from build123d import *

# Parameters (mm, degrees)
SKETCH1_W           = 120
SKETCH1_H           = 110
BOSS_EXTRUDE1_DEPTH = 2.5
SKETCH2_R           = 14.5
CUT_EXTRUDE1_DEPTH  = 4
SKETCH3_R           = 20
CUT_EXTRUDE2_DEPTH  = 10
SKETCH5_R           = 1.6
CUT_EXTRUDE5_DEPTH  = 10
CUT_EXTRUDE6_DEPTH  = 10
SKETCH8_W           = 5
SKETCH8_H           = 10
SKETCH8_W_2         = 10
SKETCH8_H_2         = 5
BOSS_EXTRUDE2_DEPTH = 14
SKETCH9_R           = 1.5
CUT_EXTRUDE7_DEPTH  = 120.910383203
SKETCH10_R          = 1.5
CUT_EXTRUDE8_DEPTH  = 5
FILLET1_R           = 2.5


with BuildPart() as part:
    # Sketch1 → Boss-Extrude1 (new body)
    with BuildSketch(Plane(origin=(0, 0, 0), x_dir=(1, 0, 0), z_dir=(0, 1, 0))):
        Rectangle(SKETCH1_W, SKETCH1_H)
    extrude(amount=BOSS_EXTRUDE1_DEPTH)

    # Sketch2 → Cut-Extrude1 (cut)
    with BuildSketch(Plane(origin=(0, 2.5, 0), x_dir=(1, 0, 0), z_dir=(0, 1, 0))):
        with Locations(Location((40, 30, 0), (0, 0, 270))):
            Circle(SKETCH2_R)
        with Locations(Location((10, 30, 0), (0, 0, 270))):
            Circle(SKETCH2_R)
        with Locations(Location((-40, -5, 0), (0, 0, 270))):
            Circle(SKETCH2_R)
        with Locations(Location((-40, -35, 0), (0, 0, 270))):
            Circle(SKETCH2_R)
    extrude(amount=-CUT_EXTRUDE1_DEPTH, mode=Mode.SUBTRACT)

    # Sketch3 → Cut-Extrude2 (cut)
    with BuildSketch(Plane(origin=(0, 2.5, 0), x_dir=(1, 0, 0), z_dir=(0, 1, 0))):
        with Locations(Location((25, -20, 0), (0, 0, 270))):
            Circle(SKETCH3_R)
    extrude(amount=-CUT_EXTRUDE2_DEPTH, mode=Mode.SUBTRACT)

    # Sketch5 → Cut-Extrude5 (cut)
    with BuildSketch(Plane(origin=(0, 2.5, 0), x_dir=(1, 0, 0), z_dir=(0, 1, 0))):
        with Locations(Location((-56, 51, 0), (0, 0, 270))):
            Circle(SKETCH5_R)
        with Locations(Location((56, 51, 0), (0, 0, 270))):
            Circle(SKETCH5_R)
        with Locations(Location((56, -51, 0), (0, 0, 270))):
            Circle(SKETCH5_R)
        with Locations(Location((-56, -51, 0), (0, 0, 270))):
            Circle(SKETCH5_R)
    extrude(amount=-CUT_EXTRUDE5_DEPTH, mode=Mode.SUBTRACT)

    # Sketch7 → Cut-Extrude6 (cut)
    with BuildSketch(Plane(origin=(0, 2.5, 0), x_dir=(1, 0, 0), z_dir=(0, 1, 0))):
        with BuildLine():
            Line((-54.5, -5), (-54.5, 0))
            ThreePointArc((-54.5, 0), (-40, 14.5), (-25.5, 0))
            Line((-25.5, 0), (-25.5, -5))
            ThreePointArc((-25.5, -5), (-40, -19.5), (-54.5, -5))
        make_face()
        with BuildLine():
            Line((10, 15.5), (5, 15.5))
            ThreePointArc((5, 15.5), (-9.5, 30), (5, 44.5))
            Line((5, 44.5), (10, 44.5))
            ThreePointArc((10, 44.5), (24.5, 30), (10, 15.5))
        make_face()
    extrude(amount=-CUT_EXTRUDE6_DEPTH, mode=Mode.SUBTRACT)

    # Sketch8 → Boss-Extrude2 (add)
    with BuildSketch(Plane(origin=(0, 2.5, 0), x_dir=(1, 0, 0), z_dir=(0, 1, 0))):
        with Locations((-17.5, -20)):
            Rectangle(SKETCH8_W, SKETCH8_H)
        with Locations((25, 50)):
            Rectangle(SKETCH8_W_2, SKETCH8_H_2)
    extrude(amount=BOSS_EXTRUDE2_DEPTH)

    # Sketch9 → Cut-Extrude7 (cut, through all)
    with BuildSketch(Plane.XY.offset(-47.5)):
        with Locations((25, 10.5)):
            Circle(SKETCH9_R)
        with BuildLine():
            Line((20, 10.5), (20, 22.099022081))
            Line((20, 22.099022081), (30, 22.099022081))
            Line((30, 22.099022081), (30, 10.5))
            ThreePointArc((30, 10.5), (25, 15.5), (20, 10.5))
        make_face()
    extrude(amount=-CUT_EXTRUDE7_DEPTH, mode=Mode.SUBTRACT)

    # Sketch10 → Cut-Extrude8 (cut)
    with BuildSketch(Plane(origin=(-15, 0, 0), x_dir=(0, 0, -1), z_dir=(1, 0, 0))):
        with Locations((-20, 10.5)):
            Circle(SKETCH10_R)
        with BuildLine():
            Line((-25, 10.5), (-25, 23.531098802))
            Line((-25, 23.531098802), (-15, 23.531098802))
            Line((-15, 23.531098802), (-15, 10.5))
            ThreePointArc((-15, 10.5), (-20, 15.5), (-25, 10.5))
        make_face()
    extrude(amount=-CUT_EXTRUDE8_DEPTH, mode=Mode.SUBTRACT)

    # Fillet1
    fillet1_edges = [part.edges().sort_by_distance(p)[0] for p in [
        (23.5, 10.5, -52.5),
        (23.5, 10.5, -47.5),
        (-20, 10.5, 21.5),
        (-15, 10.5, 21.5),
    ]]
    fillet(fillet1_edges, radius=FILLET1_R - 0.0001)  # a hair under: the kernel refuses the full size


solid = part.part
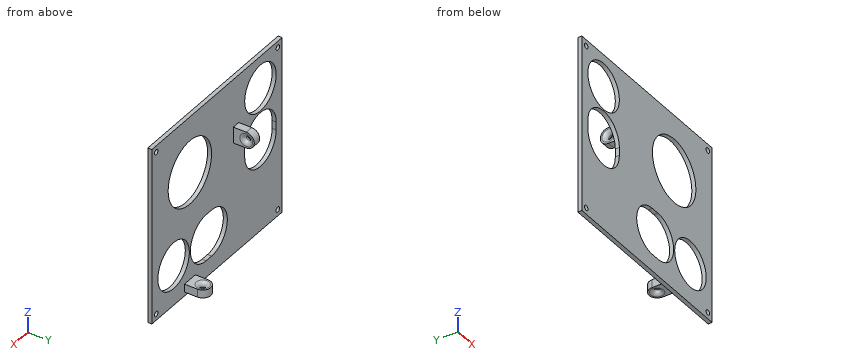
The listing builds one solid part. Answer for the finished solid, in the listing's coordinates (mm). Coordinates: 2 decimals unless noted, no trailing zeros. Loops run counter-clockwise (first coordinate to the right, second up) from the corner with the lowest first, then second, coordinate; pieces in that order, holes last. Notation, with made-up numbers: (25.5, 63) -> (71.5, 63) arc R18 cw to (71.5, 79) -> close; hole circle Ø5 at (54, -4). An arc over 180 degrees is marked (long way). Answer in a Markdown table with one row per item. Add a question column.
1. The part is cut by section B-B, the plane x = 35.5. Write down the section's boundary in (y, z).
2. Flat-ended cylindrical pins translate along their axes: P1, Ø1, axis at y = 5, z = 15, coming from the -X side; P2, Ø2.5, axis at x = -18.5, y = 8, coming from the -Z side; P3, Ø3.5, axis at y = 10.5, z = 20, coming from the +X side. Find the tip coordinate at first contact, or state that the pin passes through.
3. Consider line 1 (X direction, y = 0.6, z = 51); line 2 (X direction, y = 1.7, z = 35); line 3 (Z direction, x = 36, y = 1). Determine where each line is inside the solid, lowest interval first. Write a range as [from, to].
4. The part is cut by section A-A, the plane z = -19.5. Write down the section's boundary in (x, y), then the cut area to 4 significant figures.
5. The part is cut by section C-C, the plane x = 3. Write down the section's boundary in (y, z).
Answer below:
| question | item | result |
|---|---|---|
| 1 | outline | (0, -55) -> (2.5, -55) -> (2.5, -43.78) -> (0, -43.78) -> close; (0, -16.22) -> (2.5, -16.22) -> (2.5, 2.98) -> (0, 2.98) -> close; (0, 37.02) -> (2.5, 37.02) -> (2.5, 55) -> (0, 55) -> close |
| 2 | P1 | x = -20 |
| 2 | P2 | z = 15 |
| 2 | P3 | x = -16.41 |
| 3 | line 1 | [-60, -57.6], [-54.4, 54.4], [57.6, 60] |
| 3 | line 2 | [-60, -54.5], [-25.5, 11.77], [38.23, 60] |
| 3 | line 3 | [-55, -43.94], [-16.06, 3.3], [36.7, 55] |
| 4 | outline | (-60, 0) -> (-5, 0) -> (-5, 2.5) -> (-60, 2.5) -> close; (20, 0) -> (30, 0) -> (30, 2.5) -> (20, 2.5) -> close; (50, 0) -> (60, 0) -> (60, 2.5) -> (50, 2.5) -> close |
| 4 | area | 187.5 mm2 |
| 5 | outline | (0, -55) -> (2.5, -55) -> (2.5, -44.36) -> (0, -44.36) -> close; (0, -15.64) -> (2.5, -15.64) -> (2.5, 55) -> (0, 55) -> close |
